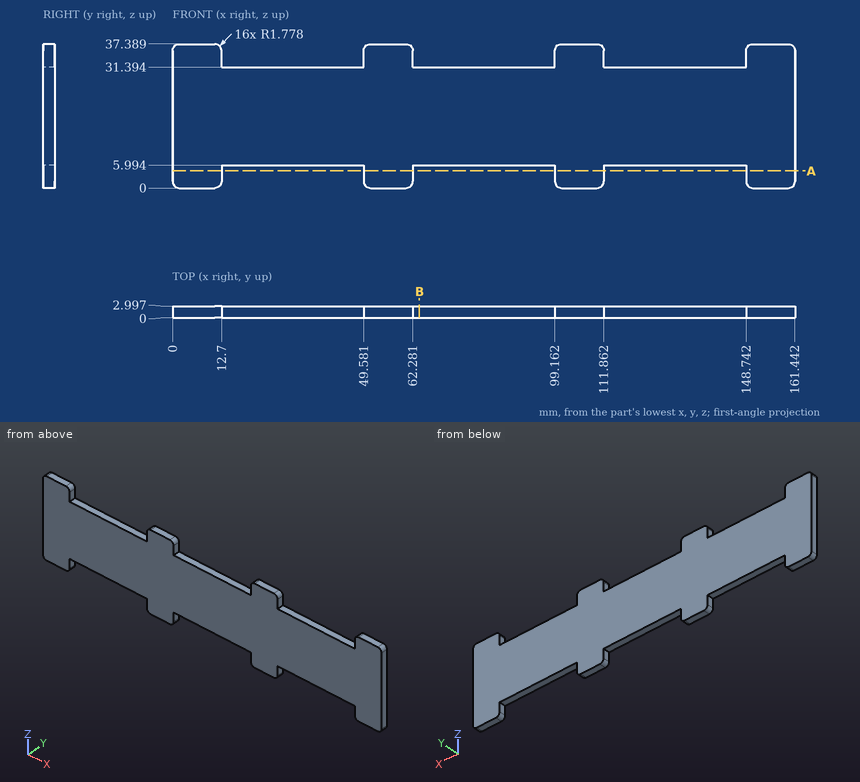
The drawing under review shows one solid part. Ordinate dimensions are in mm from its lowest x, y, z. Coordinates: 2 decimals unless noted, no trailing zeros. Loops run counter-clockwise (first coordinate to the right, second up) from the corner with the lowest first, then second, coordinate; pieces in that order, holes last. Notation, with made-up numbers: (10, 61.25) -> (64, 61.25) arc R25 ccw to (64, 75.25) -> close; hole circle Ø8 at (86.25, 40). An arc over 180 degrees is marked (long way). Answer as a JSON object with one key per item and string values.
Q1. Take a section at A-A on z = 4.5. Give the boundary of the cut face in (x, y), plus the area to 3 significant figures.
Answer block:
{"outline": "(0, 0) -> (12.7, 0) -> (12.7, 3) -> (0, 3) -> close; (49.58, 0) -> (62.28, 0) -> (62.28, 3) -> (49.58, 3) -> close; (99.16, 0) -> (111.86, 0) -> (111.86, 3) -> (99.16, 3) -> close; (148.74, 0) -> (161.44, 0) -> (161.44, 3) -> (148.74, 3) -> close", "area": "152 mm^2"}
Q2. To check wall thickness, follow L1, parallel to X at y = 2.8, z = 2; L2, parallel to Z at x = 91.5, y = 2.8 (1 decimal). State the ranges of each line that lie inside material, in increasing order.
Answer block:
{"L1": "x = 0 to 12.7, 49.58 to 62.28, 99.16 to 111.86, 148.74 to 161.44", "L2": "z = 6 to 31.4"}
Q3. Take a section at B-B on x = 64. Give the boundary of the cut face in (y, z) (1 decimal).
Answer block:
{"outline": "(0, 6) -> (3, 6) -> (3, 31.4) -> (0, 31.4) -> close"}
Q4. Clearance check with flat-ended pins moving along their axes: pin 1 Ø1.5 at (x, y) = (28.5, 1) entering from -Z; pin 2 Ø1.5 at (x, y) = (32.5, 2) entering from +Z. State where each tip first meets the part, or that it passes through.
Answer block:
{"pin 1": "stops at z = 5.99", "pin 2": "stops at z = 31.39"}
